Verification items for the finished model (mm, model axes). Coordinates: 2 decimals unless noted, no trailing zeros. Loops run counter-clockwise (first coordinate to the right, second up) from the corner with the lowest first, then second, coordinate; pieces in that order, holes last. Notation, with made-up numbers: (-17.75, -14) - (24.25, -14) arc R15 ccw to (24.25, -8) - close; hole circle Ø11 at (24, 41.25). An arc over 180 degrees is marked (long way). Answer as CSV lines item,"result". Start each with the question number.
1. Gauge pin test, flat ends, axial feed: P1, Ø7.5, axis at y = -12.7, z = 0, coming from the -X side; P2, Ø4, axis at y = -11.5, z = -0.5, coming from the +X side. Record the tip position at first contact, or that the pin passes through.
2. Material ranges on line 1 (Z direction, x = 200.25, y = -12.7); line 2 (X direction, y = -11.75, z = -5), recorded low to high. Write a range as [from, to].
3. Cross-section at B-B (z = 0). Enter the section's corners in (x, y).
4. Cross-section at A-A (y = -12.7). Enter the section's corners in (x, z), plus the area to 3 significant figures.
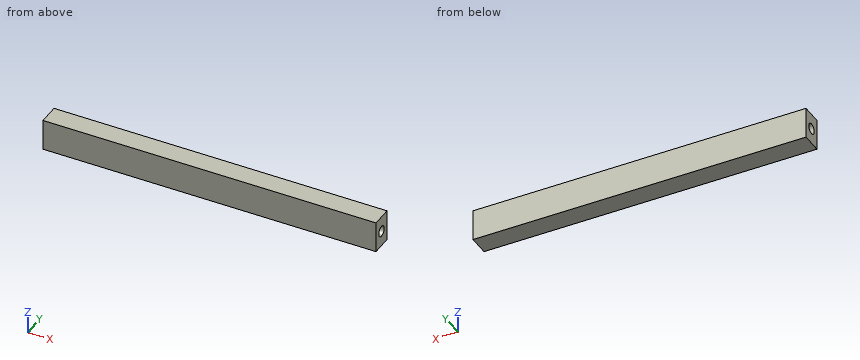
```python
from build123d import *

# Parameters (mm, degrees)
F0_W     = 406.4
F0_H     = 38.1
F1_DEPTH = 25.4
F2_R     = 6.35
F3_DEPTH = 12.7
F4_R     = 6.35
F5_DEPTH = 12.7


with BuildPart() as f1:
    # F0 (on Front) → F1 (new body)
    with BuildSketch(Plane.XZ):
        Rectangle(F0_W, F0_H)
    extrude(amount=F1_DEPTH)

    # F2 (on face) → F3 (cut)
    with BuildSketch(Plane(origin=(-203.2, 0, 0), x_dir=(0, -1, 0), z_dir=(-1, 0, 0))):
        with Locations((12.7, 0)):
            Circle(F2_R)
    extrude(amount=-F3_DEPTH, mode=Mode.SUBTRACT)

    # F4 (on face) → F5 (cut)
    with BuildSketch(Plane.YZ.offset(203.2)):
        with Locations((-12.7, 0)):
            Circle(F4_R)
    extrude(amount=-F5_DEPTH, mode=Mode.SUBTRACT)


solid = f1.part
```
Values follow:
1,P1,"stops at x = -190.5"
1,P2,"stops at x = 190.5"
2,line 1,"z = [-19.05, -6.35], [6.35, 19.05]"
2,line 2,"x = [-190.5, 190.5]"
3,outline,"(-203.2, -25.4) - (203.2, -25.4) - (203.2, -19.05) - (190.5, -19.05) - (190.5, -6.35) - (203.2, -6.35) - (203.2, 0) - (-203.2, 0) - (-203.2, -6.35) - (-190.5, -6.35) - (-190.5, -19.05) - (-203.2, -19.05) - close"
4,outline,"(-203.2, -19.05) - (203.2, -19.05) - (203.2, -6.35) - (190.5, -6.35) - (190.5, 6.35) - (203.2, 6.35) - (203.2, 19.05) - (-203.2, 19.05) - (-203.2, 6.35) - (-190.5, 6.35) - (-190.5, -6.35) - (-203.2, -6.35) - close"
4,area,"15,200 mm²"
